```python
from build123d import *

# Parameters (mm, degrees)
SKETCH2_W           = 120
SKETCH2_H           = 120
BOSS_EXTRUDE1_DEPTH = 9.525
CUT_EXTRUDE1_START  = -10.525
CUT_EXTRUDE1_DEPTH  = 11.525
CIRPATTERN1_COUNT   = 4
FILLET1_R           = 9.525


with BuildPart() as part:
    # Sketch2 → Boss-Extrude1 (new body)
    with BuildSketch(Plane.XY):
        Rectangle(SKETCH2_W, SKETCH2_H)
    extrude(amount=BOSS_EXTRUDE1_DEPTH)

    # Sketch3 → Cut-Extrude1 (cut)
    with BuildSketch(Plane.XY.offset(9.525).offset(CUT_EXTRUDE1_START)):
        with BuildLine():
            Line((-47.575330847, 52.424669153), (-35.125330847, 39.974669153))
            ThreePointArc((-35.125330847, 39.974669153), (-35.125330847, 35.125330847), (-39.974669153, 35.125330847))
            Line((-39.974669153, 35.125330847), (-52.424669153, 47.575330847))
            ThreePointArc((-52.424669153, 47.575330847), (-52.424669153, 52.424669153), (-47.575330847, 52.424669153))
        make_face()
    cut_extrude1 = extrude(amount=CUT_EXTRUDE1_DEPTH, mode=Mode.SUBTRACT)

    # CirPattern1: Cut-Extrude1 ×4 about axis
    cirpattern1_axis = Axis((0, 0, 0), (0, 0, 1))
    for i in range(1, CIRPATTERN1_COUNT):
        add(cut_extrude1.rotate(cirpattern1_axis, i * 360 / CIRPATTERN1_COUNT), mode=Mode.SUBTRACT)

    # Fillet1
    fillet1_edges = [part.edges().sort_by_distance(p)[0] for p in [
        (60, -60, 4.7625),
        (-60, -60, 4.7625),
        (-60, 60, 4.7625),
        (60, 60, 4.7625),
    ]]
    fillet(fillet1_edges, radius=FILLET1_R)


solid = part.part
```
Input: part model. Units: mm. Frame: model coordinates. A direction names the side the tool comes from. Coordinates: 2 decimals unless noted, no trailing zeros. Loops run counter-clockwise (first coordinate to the right, second up) from the corner with the lowest first, then second, coordinate; pieces in that order, holes last. Notation, with made-up numbers: (30, 66.5) - (45, 66.5) arc R32 cw to (45, 102.5) - close; hole circle Ø3 at (-22.75, -9.5). An arc over 180 degrees is marked (long way). Answer in a Markdown table with one row per item.
(1) Material intervals for L1, parallel to Y at x = 38, z = 7.25; L2, parallel to X at y = 48, z = 4; L3, parallel to Y at x = -46.5, z = 6.75, sorted ascending. Write a range as from..to.
Model answer:
| item | result |
|---|---|
| L1 | y = -60..-42.85, -34.15..34.15, 42.85..60 |
| L2 | x = -60..-52.79, -43.15..43.15, 52.79..60 |
| L3 | y = -60..-51.35, -41.65..41.65, 51.35..60 |
(2) Set-up query: faces 5 (the face through (-57.28, 57.14, 4.83)), 6 (the face through (-41.26, -46.11, 4.7)). Return all of +Z, -Z, +X, -X, +Y, -Y with unobstructed straight access to the full face (end or side cutting, diameter ignored); none if empty.
Model answer:
| item | result |
|---|---|
| face 5 | +Z, -Z, -X, +Y |
| face 6 | +Z, -Z |
(3) Cut plane A-A on z = 1.5. Output: boundary loops of the cut face in (x, y) (3 decimals), plus the area to 3 significant figures.
Model answer:
| item | result |
|---|---|
| outline | (-60, -50.475) arc R9.525 ccw to (-50.475, -60) - (50.475, -60) arc R9.525 ccw to (60, -50.475) - (60, 50.475) arc R9.525 ccw to (50.475, 60) - (-50.475, 60) arc R9.525 ccw to (-60, 50.475) - close; hole (-52.425, -47.575) arc R3.429 ccw to (-47.575, -52.425) - (-35.125, -39.975) arc R3.429 ccw to (-39.975, -35.125) - close; hole (-52.425, 47.575) - (-39.975, 35.125) arc R3.429 ccw to (-35.125, 39.975) - (-47.575, 52.425) arc R3.429 ccw to start; hole (35.125, -39.975) - (47.575, -52.425) arc R3.429 ccw to (52.425, -47.575) - (39.975, -35.125) arc R3.429 ccw to start; hole (35.125, 39.975) arc R3.429 ccw to (39.975, 35.125) - (52.425, 47.575) arc R3.429 ccw to (47.575, 52.425) - close |
| area | 13,700 mm² |
(4) Cut plane B-B on x = -37.55. Output: boundary loops of the cut face in (y, z) (3 decimals), plus the area to 3 significant figures.
Model answer:
| item | result |
|---|---|
| outline | (-60, 0) - (-42.399, 0) - (-42.399, 9.525) - (-60, 9.525) - close; (-34.121, 0) - (34.121, 0) - (34.121, 9.525) - (-34.121, 9.525) - close; (42.399, 0) - (60, 0) - (60, 9.525) - (42.399, 9.525) - close |
| area | 985 mm² |
(5) Mould query, pull axis Y, two halves, no side actions, for faces 1 (the face through (41.44, -46.29, 4.7)), 2 (the face through (-60, -1, 5)), 3 (the face through (-52.37, -52.48, 4.7)), 4 (the face through (57.14, -57.28, 4.83)). Classes: pulls with the +Y half, pulls with the -Y half, needs draft (parallel to the pull), parting line crosses it, or undercut.
Model answer:
| item | result |
|---|---|
| face 1 | undercut |
| face 2 | needs draft |
| face 3 | undercut |
| face 4 | pulls with the -Y half |
(6) Cut plane C-C on y = -45. Output: boundary loops of the cut face in (x, z) (3 decimals).
Model answer:
| item | result |
|---|---|
| outline | (-60, 0) - (-49.849, 0) - (-49.849, 9.525) - (-60, 9.525) - close; (-40.151, 0) - (40.151, 0) - (40.151, 9.525) - (-40.151, 9.525) - close; (49.849, 0) - (60, 0) - (60, 9.525) - (49.849, 9.525) - close |
